```python
from build123d import *

# Parameters (mm, degrees)
SZKIC2_R                    = 1.15000024
DODANIE_WYCI_GNI_CIE1_DEPTH = 1.5
DODANIE_WYCI_GNI_CIE2_DEPTH = 5
ZAOKR_GLENIE1_R             = 1


with BuildPart() as part:
    # Szkic2 → Dodanie-wyciągnięcie1 (new body)
    with BuildSketch(Plane(origin=(0, 0.9903587, 0), x_dir=(1, 0, 0), z_dir=(0, 1, 0))):
        with BuildLine():
            Line((-173.537057861, -25.629454659), (-177.980234802, -25.600470859))
            Line((-177.980234802, -25.600470859), (-179.465273063, -25.389138502))
            Line((-179.465273063, -25.389138502), (-179.875270484, -28.27020162))
            Line((-179.875270484, -28.27020162), (-180.220882829, -31.315847433))
            Line((-180.220882829, -31.315847433), (-180.496294073, -34.480041019))
            Line((-180.496294073, -34.480041019), (-180.693629515, -37.735565991))
            Line((-180.693629515, -37.735565991), (-180.810996631, -41.053218548))
            Line((-180.810996631, -41.053218548), (-180.844357588, -44.770440674))
            Line((-180.844357588, -44.770440674), (-180.776598606, -48.479996177))
            Line((-180.776598606, -48.479996177), (-180.606637328, -52.137204019))
            Line((-180.606637328, -52.137204019), (-180.340406733, -55.699429047))
            Line((-180.340406733, -55.699429047), (-179.981756968, -59.127877551))
            Line((-179.981756968, -59.127877551), (-179.544751696, -62.365140152))
            Line((-179.544751696, -62.365140152), (-178.058234871, -62.164471942))
            Line((-178.058234871, -62.164471942), (-173.603659928, -62.571167494))
            ThreePointArc((-173.603659928, -62.571167494), (-173.024806006, -62.44819003), (-172.616824171, -62.019533826))
            Line((-172.616824171, -62.019533826), (-172.326234878, -61.433471042))
            Line((-172.326234878, -61.433471042), (-171.806234897, -61.378472644))
            Line((-171.806234897, -61.378472644), (-171.309234799, -61.217471439))
            Line((-171.309234799, -61.217471439), (-170.856234968, -60.956471759))
            Line((-170.856234968, -60.956471759), (-170.468234957, -60.606471377))
            Line((-170.468234957, -60.606471377), (-170.161234797, -60.183471042))
            Line((-170.161234797, -60.183471042), (-169.948234976, -59.706471759))
            Line((-169.948234976, -59.706471759), (-169.840234936, -59.194472629))
            Line((-169.840234936, -59.194472629), (-169.840234936, -58.672471362))
            Line((-169.840234936, -58.672471362), (-169.948234976, -58.160472232))
            Line((-169.948234976, -58.160472232), (-170.161234797, -57.683471042))
            Line((-170.161234797, -57.683471042), (-170.468234957, -57.260472613))
            Line((-170.468234957, -57.260472613), (-170.856234968, -56.910472232))
            Line((-170.856234968, -56.910472232), (-171.309234799, -56.649472552))
            Line((-171.309234799, -56.649472552), (-171.806234897, -56.488471347))
            Line((-171.806234897, -56.488471347), (-172.326234878, -56.433471042))
            Line((-172.326234878, -56.433471042), (-173.590153384, -56.649472552))
            Line((-173.590153384, -56.649472552), (-174.035645958, -58.160472232))
            Line((-174.035645958, -58.160472232), (-174.223992711, -58.263046011))
            Line((-174.223992711, -58.263046011), (-177.48282769, -58.263046011))
            ThreePointArc((-177.48282769, -58.263046011), (-178.091581224, -58.056405409), (-178.448748365, -57.52188428))
            Line((-178.448748365, -57.52188428), (-178.765053408, -56.341511761))
            Line((-178.765053408, -56.341511761), (-178.846234978, -55.565471011))
            Line((-178.846234978, -55.565471011), (-179.109234989, -52.046471912))
            Line((-179.109234989, -52.046471912), (-179.277234734, -48.43147214))
            Line((-179.277234734, -48.43147214), (-179.344234646, -44.763472873))
            Line((-179.344234646, -44.763472873), (-179.311234654, -41.08647092))
            Line((-179.311234654, -41.08647092), (-179.195234955, -37.807471591))
            Line((-179.195234955, -37.807471591), (-179.000234783, -34.590472537))
            Line((-179.000234783, -34.590472537), (-178.728234947, -31.465472537))
            Line((-178.728234947, -31.465472537), (-178.700062197, -31.217205306))
            ThreePointArc((-178.700062197, -31.217205306), (-178.372489594, -30.58405239), (-177.706439248, -30.329959177))
            Line((-177.706439248, -30.329959177), (-174.112522963, -30.329959177))
            Line((-174.112522963, -30.329959177), (-174.022657546, -31.208577866))
            ThreePointArc((-174.022657546, -31.208577866), (-173.436715177, -32.019422034), (-172.441579371, -31.91694544))
            Line((-172.441579371, -31.91694544), (-172.326234878, -31.833472568))
            Line((-172.326234878, -31.833472568), (-171.806234897, -31.778472262))
            Line((-171.806234897, -31.778472262), (-171.309234799, -31.617472964))
            Line((-171.309234799, -31.617472964), (-170.856234968, -31.356471377))
            Line((-170.856234968, -31.356471377), (-170.468234957, -31.006472903))
            Line((-170.468234957, -31.006472903), (-170.161234797, -30.583472568))
            Line((-170.161234797, -30.583472568), (-169.948234976, -30.106471377))
            Line((-169.948234976, -30.106471377), (-169.840234936, -29.59447034))
            Line((-169.840234936, -29.59447034), (-169.840234936, -29.072470981))
            Line((-169.840234936, -29.072470981), (-169.948234976, -28.560469943))
            Line((-169.948234976, -28.560469943), (-170.161234797, -28.083472568))
            Line((-170.161234797, -28.083472568), (-170.468234957, -27.660472232))
            Line((-170.468234957, -27.660472232), (-170.856234968, -27.310469943))
            Line((-170.856234968, -27.310469943), (-171.309234799, -27.049472171))
            Line((-171.309234799, -27.049472171), (-171.806234897, -26.888472873))
            Line((-171.806234897, -26.888472873), (-172.326234878, -26.833472568))
            Line((-172.326234878, -26.833472568), (-172.647665436, -26.185208875))
            ThreePointArc((-172.647665436, -26.185208875), (-173.013661572, -25.781385351), (-173.537057861, -25.629454659))
        make_face()
        with Locations((-172.326039002, -29.333481885)):
            Circle(SZKIC2_R, mode=Mode.SUBTRACT)
        with Locations((-172.326039002, -58.933463325)):
            Circle(SZKIC2_R, mode=Mode.SUBTRACT)
    extrude(amount=DODANIE_WYCI_GNI_CIE1_DEPTH)

    # Szkic3 → Dodanie-wyciągnięcie2 (add)
    with BuildSketch(Plane.XZ.offset(-0.9903587)):
        Polygon((-178.765053408, 56.341511761), (-178.058234871, 62.164471942), (-179.544751696, 62.365140152), (-179.981756968, 59.127877551), (-180.340406733, 55.699429047), (-180.606637328, 52.137204019), (-180.776598606, 48.479996177), (-180.844357588, 44.770440674), (-180.810996631, 41.053218548), (-180.693629515, 37.735565991), (-180.496294073, 34.480041019), (-180.220882829, 31.315847433), (-179.875270484, 28.27020162), (-179.465273063, 25.389138502), (-177.980234802, 25.600470859), (-178.728234947, 31.465472537), (-179.000234783, 34.590472537), (-179.195234955, 37.807471591), (-179.311234654, 41.08647092), (-179.344234646, 44.763472873), (-179.277234734, 48.43147214), (-179.109234989, 52.046471912), (-178.846234978, 55.565471011), align=None)
    extrude(amount=DODANIE_WYCI_GNI_CIE2_DEPTH)

    # Zaokrąglenie1
    zaokr_glenie1_edges = [part.edges().sort_by_distance(p)[0] for p in [
        (-178.722753933, -4.0096413, 25.49480468),
        (-178.801493283, -4.0096413, 62.264806047),
    ]]
    fillet(zaokr_glenie1_edges, radius=ZAOKR_GLENIE1_R)


solid = part.part
```
The listing builds one solid part. Answer for the finished solid, in the listing's coordinates (mm). A direction names the side the tool comes from. Give positions to 0.01 mm unless a question says otherwise; leave off trailing zeros. Order: outer loops, then holes, each group sorted by start corner. A loop starts at its lowest first (then second) coordinate and runs counter-clockwise, first axis right, second up. Notation, with made-up numbers: (19, 86) -> (31, 86) arc R17 cw to (31, 118) -> close; hole circle Ø4 at (-12, 21.5). An arc over 180 degrees is marked (long way). Answer as a JSON object with one key per item and string values. Group by question number.
Item 1: A tool of negligible diameter and unlimited length cuts with its end or side. For faces 4 (the flat face through (-176, 2, 30.33)), 5 (the flat face through (-180, -4.01, 44)), from which of +Z, -Z, +X, -X, +Y, -Y can it reach the whole face along a straight path? Write none if from no direction.
Item 2: The part is cut by section B-B on x = -177. Write down the section's boundary in (y, z), and give its area (3 significant figures).
Item 3: The part is cut by section C-C on z = 35. Write down the section's boundary in (x, y).
Item 4: Determine the mould class of faces 1 (the flat face through (-174, 0.99, 29)), 2 (the flat face through (-179.096, -0.714, 36.176)), 3 (the flat face through (-174.07, 1.73, 30.76)) for opening direction X: pulls with the +X half, pulls with the -X half, needs draft (parallel to the pull), parting line crosses it, or undercut.
Item 5: The part is cut by section A-A on x = -175.5. Write down the section's boundary in (y, z), and give its area (3 significant figures).
Item 6: Consider L1, parallel to Y at x = -175.5, z = 28.5; L2, parallel to X at y = -0.75, z = 61; L3, parallel to X at y = -2.5, z = 45.5. Determine where each line is inside the solid, lowest interval first. Write a range as from..to.
Item 7: The part is cut by section D-D on z = 48. Write down the section's boundary in (x, y), and give its area (3 significant figures).
Item 8: Flat-ended cylindrical pins translate along their axes: pin 1 (1 mm diameter, centred on x = -172.5, y = 1.5, fed in from +Z); pin 2 (3 mm diameter, centred on x = -172.33, z = 29.33, fed in from +Y); pin 3 (5 mm diameter, centred on x = -172.5, z = 28.5, fed in from -Y). Find the tip coordinate at first contact, or state that the pin passes through.
Result set:
{
 "1": {"face 4": "+Y, -Y", "face 5": "+Z, -Z, +X, -X, -Y"},
 "2": {"outline": "(0.99, 25.61) -> (2.49, 25.61) -> (2.49, 30.33) -> (0.99, 30.33) -> close; (0.99, 58.26) -> (2.49, 58.26) -> (2.49, 62.26) -> (0.99, 62.26) -> close", "area": "13.1 mm²"},
 "3": {"outline": "(-180.53, -4.01) -> (-179.03, -4.01) -> (-179.03, 2.49) -> (-180.53, 2.49) -> close"},
 "4": {"face 1": "needs draft", "face 2": "pulls with the +X half", "face 3": "undercut"},
 "5": {"outline": "(0.99, 25.62) -> (2.49, 25.62) -> (2.49, 30.33) -> (0.99, 30.33) -> close; (0.99, 58.26) -> (2.49, 58.26) -> (2.49, 62.4) -> (0.99, 62.4) -> close", "area": "13.3 mm²"},
 "6": {"L1": "0.99..2.49", "L2": "-179.73..-178.2", "L3": "-180.83..-179.33"},
 "7": {"outline": "(-180.79, -4.01) -> (-179.29, -4.01) -> (-179.29, 2.49) -> (-180.79, 2.49) -> close", "area": "9.75 mm²"},
 "8": {"pin 1": "z = 62.43", "pin 2": "y = 2.49", "pin 3": "y = 0.99"}
}
